Job drawing, mm, ordinate dimensions from the low corner. One solid piece. Give positions to 0.01 mm unless a question says otherwise; leave off trailing zeros. Loops run counter-clockwise (first coordinate to the right, second up) from the corner with the lowest first, then second, coordinate; pieces in that order, holes last. Notation, with made-up numbers: M 54.5,-5 L 92.5,-5 A21 cw 92.5,7 Z; hole C -4,-35 d1. An arc over 180 degrees is marked long. Answer as CSV lines item,"result".
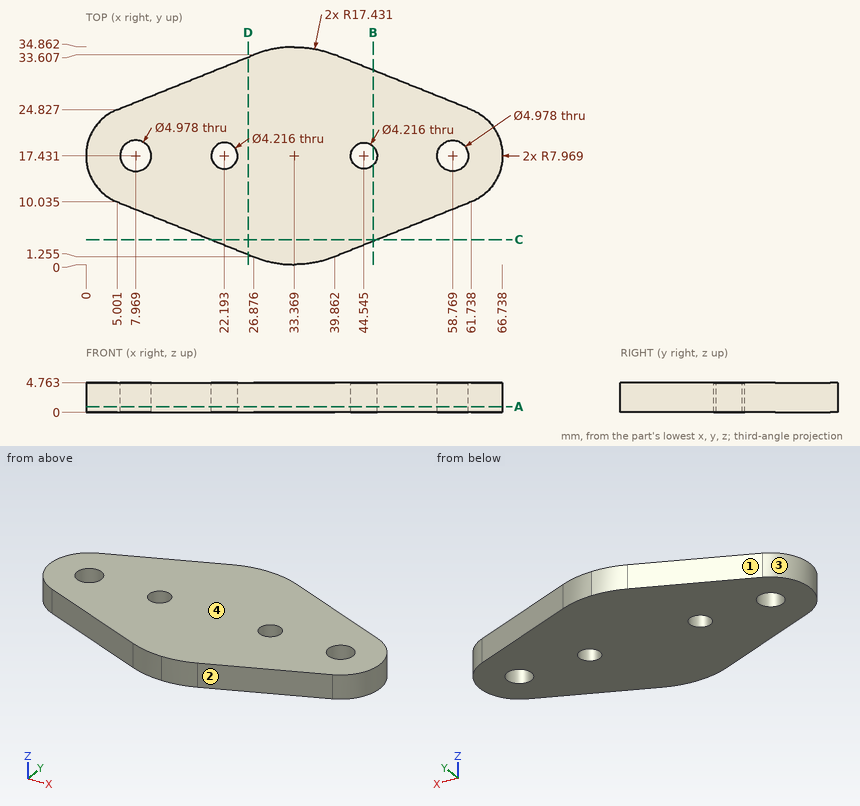
1) Mould opens along Y. For the marked faces 1, 2, 3 and 4 say: +Y half, -Y half, draft (parallel to the pull), parting line (faces both ways), or undercut.
Answer below:
face 1,"+Y half"
face 2,"-Y half"
face 3,"parting line"
face 4,"draft"
2) Drill centre lines: line 1 (X direction, y = 17.5, z = 0.8); line 2 (X direction, y = 18, z = 4.1) (1 decimal); line 3 (Y direction, x = 9, z = 2.75) (1 decimal). Where is each one in solid material? Low to high. Write a range as from..to.
Answer below:
line 1,"x = 0..5.48, 10.46..20.09, 24.3..42.44, 46.65..56.28, 61.26..66.74"
line 2,"x = 0..5.5, 10.4..20.2, 24.2..42.5, 46.6..56.3, 61.2..66.7"
line 3,"y = 8.4..15.2, 19.7..26.4"
3) Band-saw the part on B-B on x = 46. Give the cut face in (y, z) (1 decimal), and give its area (3 significant figures).
Answer below:
outline,"M 3.7,0 L 15.9,0 L 15.9,4.8 L 3.7,4.8 Z; M 19,0 L 31.1,0 L 31.1,4.8 L 19,4.8 Z"
area,"116 mm^2"
4) Band-saw the part on C-C on y = 4. Give the cut face in (x, z).
Answer below:
outline,"M 20.04,0 L 46.7,0 L 46.7,4.76 L 20.04,4.76 Z"
5) Flat gauge pins, fed straight in: pin 1 (4 mm diameter, centred on x = 44.55, y = 17.43, fed in from +Z); pin 2 (1 mm diameter, centred on y = 7.5, z = 2, fed in from -X) (1 decimal). Where does each tip first touch, or does it go through?
Answer below:
pin 1,"passes through"
pin 2,"stops at x = 10.1"
6) Band-saw the part on A-A on z = 0.9. Give the cut face in (x, y) (1 decimal), and give its area (3 significant figures).
Answer below:
outline,"M 5,10 L 26.9,1.3 A17.4 ccw 33.4,0 A17.4 ccw 39.9,1.3 L 61.7,10 A8 ccw 61.7,24.8 L 39.9,33.6 A17.4 ccw 33.4,34.9 A17.4 ccw 26.9,33.6 L 5,24.8 A8 ccw Z; hole C 8,17.4 d5; hole C 22.2,17.4 d4.2; hole C 44.5,17.4 d4.2; hole C 58.8,17.4 d5"
area,"1,510 mm^2"
7) Band-saw the part on D-D on x = 26. Give the cut face in (y, z) (1 decimal).
Answer below:
outline,"M 1.6,0 L 33.3,0 L 33.3,4.8 L 1.6,4.8 Z"
